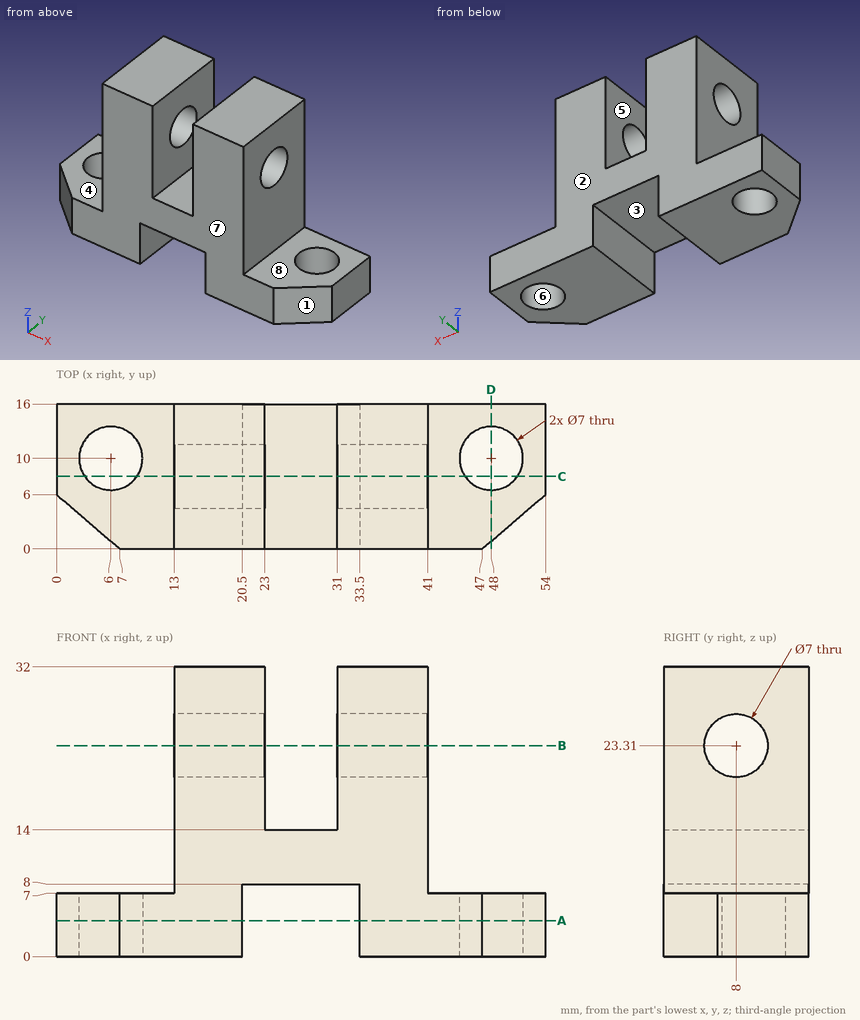
Could you check a few things on this drawing? It's one solid part, dimensions in mm from its lowest x, y, z. A direction names the side the tool comes from. Coordinates: 2 decimals unless noted, no trailing zeros. Loops run counter-clockwise (first coordinate to the right, second up) from the corner with the lowest first, then second, coordinate; pieces in that order, holes last.
1. I need wall thicknesses on L1, parallel to X at y = 2, z = 24.5; L2, parallel to Z at x = 15.75, y = 8; L3, parallel to X at y = 11.5, z = 4. Which ranges of each line are inside material? Lowest first, please.
2. Imagine slicing it at D-D (x = 48). Please give me the cut outline in (y, z), and give its area (3 significant figures).
3. For P1, Ø6, axis at x = 45.5, z = 13, coming from the +Y side; P2, Ø4, axis at x = 27, y = 6.5, coming from the +Z side; P3, Ø5, axis at y = 12.5, z = 27, coming from the +X side; P4, Ø4, axis at x = 6.5, y = 3.5, coming from the +Z side, each with a flat end and sliding along its axis, tell me the tip position at first contact or that it passes through.
4. For the marked faces 4, 5, 6, 7 and 8, which set-ups out of +Z, -Z, +X, -X, +Y, -Y let a thin tool reach every point of the face, with its end or its side?
5. We'd pull the mould along X, two halves only. Please class the marked faces 1, 2 and 3: released by +X, released by -X, zero draft, split by the parting line, or undercut.
6. Imagine slicing it at A-A (z = 4). Please give me the cut outline in (x, y).
7. Imagine slicing it at C-C (y = 8). Give the number of separate pieces and of enclosed holes in the cut face, and give its area (3 significant figures).
8. Imagine slicing it at B-B (z = 23.31). Please give me the cut outline in (x, y), and give its area (3 significant figures).
Computed values:
1. L1: x = 13 to 23, 31 to 41
1. L2: z = 0 to 19.81, 26.81 to 32
1. L3: x = 0 to 2.84, 9.16 to 20.5, 33.5 to 44.84, 51.16 to 54
2. outline: (0.86, 0) - (6.5, 0) - (6.5, 7) - (0.86, 7) - close; (13.5, 0) - (16, 0) - (16, 7) - (13.5, 7) - close
2. area: 57.0 mm2
3. P1: passes through
3. P2: stops at z = 14
3. P3: stops at x = 41
3. P4: stops at z = 7
4. face 4: +Z, -X, +Y, -Y
4. face 5: +Z, +Y, -Y
4. face 6: +Z, -Z
4. face 7: +Z, -Z, +X, -X, -Y
4. face 8: +Z, +X, +Y, -Y
5. face 1: released by +X
5. face 2: zero draft
5. face 3: undercut
6. outline: (0, 6) - (7, 0) - (20.5, 0) - (20.5, 16) - (0, 16) - close; (33.5, 0) - (47, 0) - (54, 6) - (54, 16) - (33.5, 16) - close; hole circle Ø7 at (6, 10); hole circle Ø7 at (48, 10)
7. separate pieces: 5
7. enclosed holes: 0
7. area: 610 mm2
8. outline: (13, 0) - (23, 0) - (23, 4.5) - (13, 4.5) - close; (13, 11.5) - (23, 11.5) - (23, 16) - (13, 16) - close; (31, 0) - (41, 0) - (41, 4.5) - (31, 4.5) - close; (31, 11.5) - (41, 11.5) - (41, 16) - (31, 16) - close
8. area: 180 mm2
